The listing builds one solid part. Answer for the finished solid, in the listing's coordinates (mm). A direction names the side the tool comes from. Round coordinates to 2 decimals unless told otherwise and drop trailing zeros. Order: outer loops, then holes, each group sorted by start corner. A loop starts at its lowest first (then second) coordinate and runs counter-clockwise, first axis right, second up. Notation, with made-up numbers: (7, 22.25) - (17, 22.25) arc R5 cw to (17, 28.25) - close; hole circle Ø1 at (27.25, -6). An arc over 180 degrees is marked (long way). One line per item, written item: value. Start each with the question number.
1. For a pull along Z with two mould halves and no side action, classify faces 3 (the cylindrical face through (1.521, 80.057, 9.513)), 4 (the flat face through (1, 74, 30)), 5 (the flat face through (1, 16, 0)) as released by +Z, released by -Z, zero draft, split by the parting line, or undercut.
2. A tool of negligible diameter and unlimited length cuts with its end or side. For faces 1 (the cylindrical face through (1.521, 1.203, 28.859)), 2 (the cylindrical face through (1.52, 73.25, 12.63)), from which of +Z, -Z, +X, -X, +Y, -Y can it reach the whole face along a straight path? Write none if from no direction.
3. Section A-A, the plane y = 45 is taken. Give the vertices of the cut face in (x, z), then the cut area to 3 significant figures.
4. Section C-C, the plane x = 0.8 is taken. Count the separate pieces of the cut face and the enclosed holes in it, then the cut area to 3 significant figures.
5. Straight lines are drawn through the part: line 1 (Z direction, x = 0.65, y = 70.5); line 2 (Y direction, x = 0.2, z = 12); line 3 (Z direction, x = 1.15, y = 86). For each, find the intervals that lie inside material, in ascending order.
6. Flat-ended cylindrical pins translate along their axes: P1, Ø2, axis at y = 10.12, z = 20, coming from the -X side; P2, Ø0.9, axis at x = 1, y = 16.5, coming from the -Z side; P3, Ø1.5, axis at x = 1.5, y = 13.5, coming from the +Z side. Find the tip coordinate at first contact, or state that the pin passes through.
7. Section B-B, the plane y = 10.12 is taken. Give the vertices of the cut face in (x, z), then the cut area to 3 significant figures.
from build123d import *

# Parameters (mm, degrees)
SKETCH_1_W          = 3
SKETCH_1_H          = 30
EXTRUDE_1_DEPTH     = 90
SKETCH_2_R          = 22.5
EXTRUDE_2_DEPTH     = 3
SKETCH_3_R          = 13
CUT_EXTRUDE_1_DEPTH = 98.546142927
HOLE_WIZARD_M31_D   = 3.4
HOLE_WIZARD_M32_D   = 3.4
FILLET_1_R          = 4
M3X0_51_D           = 2.5
CUT_EXTRUDE_2_DEPTH = 98.546142927
FILLET_2_R          = 2


with BuildPart() as part:
    # Эскиз1 → Бобышка-Вытянуть1 (new body)
    with BuildSketch(Plane(origin=(0, 0, 0), x_dir=(1, 0, 0), z_dir=(0, 1, 0))):
        with Locations((1.5, -15)):
            Rectangle(SKETCH_1_W, SKETCH_1_H)
    extrude(amount=EXTRUDE_1_DEPTH)

    # Эскиз2 → Бобышка-Вытянуть2 (add)
    with BuildSketch(Plane.ZY):
        with Locations((15, 45)):
            Circle(SKETCH_2_R)
    extrude(amount=-EXTRUDE_2_DEPTH)

    # Эскиз3 → Вырез-Вытянуть1 (cut, through all)
    with BuildSketch(Plane.ZY):
        with Locations((15, 45)):
            Circle(SKETCH_3_R)
    extrude(amount=-CUT_EXTRUDE_1_DEPTH, mode=Mode.SUBTRACT)

    # Отверстие с зазором M31 (through all)
    with Locations(Plane(origin=(3, -25.024735225, 7.262908886), x_dir=(0, 0, 1), z_dir=(1, 0, 0))):
        with Locations((21.348896652, -83.636540763), (-5.874714424, -83.636540763), (-5.874714424, -56.412929688), (21.348896652, -56.412929688)):
            Hole(HOLE_WIZARD_M31_D / 2)

    # Отверстие с зазором M32 (through all)
    with Locations(Plane(origin=(3, 0, 0), x_dir=(0, 0, -1), z_dir=(1, 0, 0))):
        with Locations((-26, 86), (-4, 86), (-4, 4), (-26, 4)):
            Hole(HOLE_WIZARD_M32_D / 2)

    # Скругление1
    fillet_1_edges = [part.edges().sort_by_distance(p)[0] for p in [
        (1.5, 90, 0),
        (1.5, 0, 0),
        (1.5, 0, 30),
        (1.5, 90, 30),
    ]]
    fillet(fillet_1_edges, radius=FILLET_1_R)

    # Отверстие обработанное метчиком M3x0.51 (through all)
    with Locations(Plane.ZY):
        with Locations((10, 60.12), (20, 60.12), (10, 10.12), (20, 10.12)):
            Hole(M3X0_51_D / 2)

    # Эскиз14 → Вырез-Вытянуть2 (cut, through all)
    with BuildSketch(Plane.ZY):
        with BuildLine():
            Line((13, 73.494171949), (13, 67.410934831))
            ThreePointArc((13, 67.410934831), (8.352708916, 66.495662847), (4, 64.627786426))
            Line((4, 64.627786426), (4, 76.769904057))
            Line((4, 76.769904057), (13, 73.494171949))
        make_face()
        with BuildLine():
            Line((17, 73.494171949), (17, 67.410934831))
            ThreePointArc((17, 67.410934831), (21.647291084, 66.495662847), (26, 64.627786426))
            Line((26, 64.627786426), (26, 76.769904057))
            Line((26, 76.769904057), (17, 73.494171949))
        make_face()
        Polygon((7.538207724, 79.738812853), (15, 77.02294257), (22.461792276, 79.738812853), (15, 86), align=None)
    extrude(amount=-CUT_EXTRUDE_2_DEPTH, mode=Mode.SUBTRACT)

    # Скругление2
    fillet_2_edges = [part.edges().sort_by_distance(p)[0] for p in [
        (1.5, 67.410934831, 13),
        (1.5, 64.627786426, 4),
        (1.5, 76.769904057, 4),
        (1.5, 73.494171949, 13),
        (1.5, 28.229490169, 0),
        (1.5, 61.770509831, 0),
        (1.5, 64.627786426, 26),
        (1.5, 67.410934831, 17),
        (1.5, 73.494171949, 17),
        (1.5, 76.769904057, 26),
        (1.5, 79.738812853, 7.538207724),
        (1.5, 86, 15),
        (1.5, 79.738812853, 22.461792276),
        (1.5, 77.02294257, 15),
        (1.5, 28.229490169, 30),
        (1.5, 61.770509831, 30),
    ]]
    fillet(fillet_2_edges, radius=FILLET_2_R)


solid = part.part
Answer list:
1. face 3: undercut
1. face 4: released by +Z
1. face 5: released by -Z
2. face 1: +Z, +X, -X, -Y
2. face 2: +X, -X
3. outline: (0, -7.5) - (3, -7.5) - (3, 2) - (0, 2) - close; (0, 28) - (3, 28) - (3, 37.5) - (0, 37.5) - close
3. area: 57.0 mm²
4. separate pieces: 1
4. enclosed holes: 16
4. area: 2,200 mm²
5. line 1: z = 0 to 4, 13 to 17, 26 to 30
5. line 2: y = 0 to 32.35, 57.65 to 67.44, 73.83 to 78.11, 83.48 to 90
5. line 3: z = 0 to 2.3, 5.7 to 24.3, 27.7 to 30
6. P1: passes through
6. P2: stops at z = 0
6. P3: stops at z = 30
7. outline: (0, 0) - (3, 0) - (3, 8.75) - (0, 8.75) - close; (0, 11.25) - (3, 11.25) - (3, 18.75) - (0, 18.75) - close; (0, 21.25) - (3, 21.25) - (3, 30) - (0, 30) - close
7. area: 75.0 mm²
